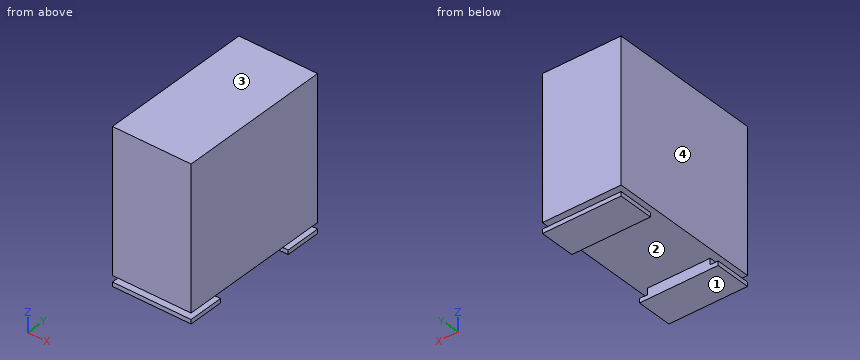
from build123d import *

# Parameters (mm, degrees)
F0_W     = 188
F0_H     = 365
F1_DEPTH = 370
F2_W     = 198
F2_H     = 25
F3_DEPTH = 188.001
F4_W     = 19.05
F4_H     = 14.84
F5_DEPTH = 370.001
F6_W     = 19.05
F6_H     = 14.84
F7_DEPTH = 188.001


with BuildPart() as f1:
    # F0 (on Front) → F1 (new body)
    with BuildSketch(Plane.XZ):
        with Locations((94, 182.5)):
            Rectangle(F0_W, F0_H)
    extrude(amount=-F1_DEPTH)

    # F2 (on face) → F3 (cut, through all)
    with BuildSketch(Plane(origin=(0, 0, 0), x_dir=(0, -1, 0), z_dir=(-1, 0, 0))):
        with Locations((-185, 12.5)):
            Rectangle(F2_W, F2_H)
    extrude(amount=-F3_DEPTH, mode=Mode.SUBTRACT)

    # F4 (on face) → F5 (cut, through all)
    with BuildSketch(Plane.XZ):
        with Locations((9.525, 17.58)):
            Rectangle(F4_W, F4_H)
        with Locations((178.475, 17.58)):
            Rectangle(F4_W, F4_H)
    extrude(amount=-F5_DEPTH, mode=Mode.SUBTRACT)

    # F6 (on face) → F7 (cut, through all)
    with BuildSketch(Plane(origin=(0, 0, 0), x_dir=(0, -1, 0), z_dir=(-1, 0, 0))):
        with Locations((-360.475, 17.58)):
            Rectangle(F6_W, F6_H)
        with Locations((-9.525, 17.58)):
            Rectangle(F6_W, F6_H)
    extrude(amount=-F7_DEPTH, mode=Mode.SUBTRACT)


solid = f1.part
Model file for the job. Use its own axes, mm. Face numbers are marked on the shaded views. Give positions to 0.01 mm unless a question says otherwise; leave off trailing zeros. Order: outer loops, then holes, each group sorted by start corner. A loop starts at its lowest first (then second) coordinate and runs counter-clockwise, first axis right, second up. Notation, with made-up numbers: M 6,-15 L 50,-15 A20 cw 50,7 Z; hole C -11.5,22.25 d2. An arc over 180 degrees is marked long. Put each result on its own line as item: value. Start each with the question number.
(1) Band-saw the part on B-B on y = 244. Give the cut face in (x, z), then the cut area to 3 significant figures.
(2) Band-saw the part on A-A on x = 120. Give the cut face in (y, z).
(3) Pull direction Z, two halves, no side cores. Call the marked faces 1, 2, 3 and 4: released by +Z, released by -Z, zero draft, split by the parting line, or undercut.
(4) Pin check, flat tips, straight feed: pin 1 Ø5 at (x, z) = (106, 267.5) entering from -Y; pin 2 Ø7.5 at (x, z) = (109.5, 18.5) entering from +Y; pin 3 Ø12 at (y, z) = (315, 16.5) entering from -X; pin 4 Ø1 at (x, y) = (19.5, 262.5) entering from -Z. Stop position of each tip, or through.
(5) Drill centre lines: L1, parallel to Z at x = 171.5, y = 345; L2, parallel to Z at x = 8.5, y = 171.5. Where is each one in solid material? Low to high. Write a range as [from, to].
Results below:
1. outline: M 0,25 L 188,25 L 188,365 L 0,365 Z
1. area: 63,900 mm2
2. outline: M 0,0 L 86,0 L 86,25 L 284,25 L 284,0 L 370,0 L 370,10.16 L 350.95,10.16 L 350.95,25 L 370,25 L 370,365 L 0,365 L 0,25 L 19.05,25 L 19.05,10.16 L 0,10.16 Z
3. face 1: released by -Z
3. face 2: undercut
3. face 3: released by +Z
3. face 4: zero draft
4. pin 1: stops at y = 0
4. pin 2: stops at y = 350.95
4. pin 3: stops at x = 19.05
4. pin 4: stops at z = 25
5. L1: z = [0, 10.16], [25, 365]
5. L2: z = [25, 365]
